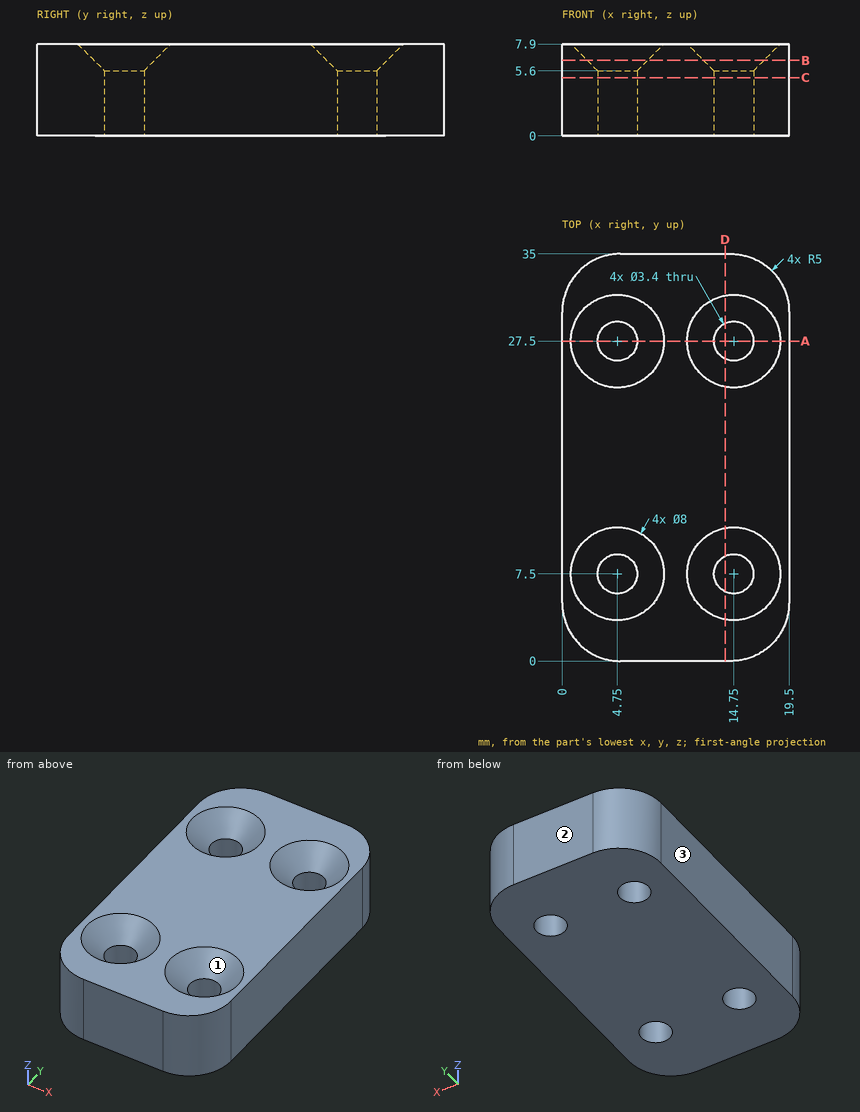
Part print with two shaded views. Sizes in mm from the minimum x, y, z corner. Coordinates: 2 decimals unless noted, no trailing zeros. Write each loop counter-clockwise with the first axis right and the second up, starting at its lowest first coordinate (ties: lowest second). Pieces come first, ordered by that corner, then holes. Notation, with made-up numbers: (66.25, 26.5) -> (88.25, 26.5) arc R17 cw to (88.25, 52.5) -> close; hole circle Ø10 at (62.5, 8.25). An arc over 180 degrees is marked (long way). Return JSON: item names as keys, results as strings. Group by question number.
Q1. Flat gauge pins, fed straight in: pin 1 (4.5 mm diameter, centred on x = 4.75, y = 7.5, fed in from +Z); pin 2 (2 mm diameter, centred on x = 14.75, y = 27.5, fed in from +Z); pin 3 (1.5 mm diameter, centred on x = 2.5, z = 5, fed in from -Y). Where does each tip first touch, or does it go through?
Q2. Cut at B-B, the plane z = 6.5. Give the cut face in (x, y), then the cut area to 3 significant figures.
Q3. Cut at C-C, the plane z = 5. Give the cut face in (x, y), then the cut area to 3 significant figures.
Q4. Cut at A-A, the plane y = 27.5. Give the cut face in (x, z).
Q5. Pull direction Y, two halves, no side cores. Call the marked faces 1, 2 and 3: released by +Y, released by -Y, zero draft, split by the parting line, or undercut.
Q6. Drill centre lines: line 1 (X direction, y = 7.5, z = 1.8); line 2 (Y direction, x = 14.75, z = 3.4); line 3 (X direction, y = 9, z = 0.5). Where is each one in solid material? Low to high.
Q7. Cut at D-D, the plane x = 14. State how many separate pieces and enclosed holes the cut face has, then the cut area to 3 significant figures.
Returned:
{
 "1": {"pin 1": "stops at z = 6.15", "pin 2": "passes through", "pin 3": "stops at y = 0.32"},
 "2": {"outline": "(0, 5) arc R5 ccw to (5, 0) -> (14.5, 0) arc R5 ccw to (19.5, 5) -> (19.5, 30) arc R5 ccw to (14.5, 35) -> (5, 35) arc R5 ccw to (0, 30) -> close; hole circle Ø5.2 at (4.75, 7.5); hole circle Ø5.2 at (4.75, 27.5); hole circle Ø5.2 at (14.75, 7.5); hole circle Ø5.2 at (14.75, 27.5)", "area": "576 mm2"},
 "3": {"outline": "(0, 5) arc R5 ccw to (5, 0) -> (14.5, 0) arc R5 ccw to (19.5, 5) -> (19.5, 30) arc R5 ccw to (14.5, 35) -> (5, 35) arc R5 ccw to (0, 30) -> close; hole circle Ø3.4 at (4.75, 7.5); hole circle Ø3.4 at (4.75, 27.5); hole circle Ø3.4 at (14.75, 7.5); hole circle Ø3.4 at (14.75, 27.5)", "area": "625 mm2"},
 "4": {"outline": "(0, 0) -> (3.05, 0) -> (3.05, 5.6) -> (0.75, 7.9) -> (0, 7.9) -> close; (6.45, 0) -> (13.05, 0) -> (13.05, 5.6) -> (10.75, 7.9) -> (8.75, 7.9) -> (6.45, 5.6) -> close; (16.45, 0) -> (19.5, 0) -> (19.5, 7.9) -> (18.75, 7.9) -> (16.45, 5.6) -> close"},
 "5": {"face 1": "undercut", "face 2": "released by +Y", "face 3": "zero draft"},
 "6": {"line 1": "x = 0 to 3.05, 6.45 to 13.05, 16.45 to 19.5", "line 2": "y = 0.01 to 5.8, 9.2 to 25.8, 29.2 to 34.99", "line 3": "x = 0 to 3.95, 5.55 to 13.95, 15.55 to 19.5"},
 "7": {"separate pieces": "3", "enclosed holes": "0", "area": "217 mm2"}
}
